For this review, take the finished solid that the model builds, in its own axes (mm). A direction names the side the tool comes from. Give positions to 0.01 mm unless a question says otherwise; leave off trailing zeros. Order: outer loops, then holes, each group sorted by start corner. A loop starts at its lowest first (then second) coordinate and runs counter-clockwise, first axis right, second up. Notation, with made-up numbers: (5, 25) - (30, 25) arc R19 cw to (30, 53) - close; hole circle Ø11 at (88, -4). An arc over 180 degrees is marked (long way). Answer as a JSON object with one key per item and string values. Group by question number.
from build123d import *

# Parameters (mm, degrees)
SKETCH1_W             = 30
SKETCH1_H             = 20
BOSS_EXTRUDE1_DEPTH   = 4
SKETCH2_R             = 4
BOSS_EXTRUDE2_DEPTH   = 3.5
M4X0_7_TAPPED_HOLE1_D = 3.3
SKETCH6_R             = 3
SKETCH6_R_2           = 1.65
BOSS_EXTRUDE3_DEPTH   = 0.5


with BuildPart() as part:
    # Sketch1 → Boss-Extrude1 (new body)
    with BuildSketch(Plane(origin=(0, 0, 0), x_dir=(1, 0, 0), z_dir=(0, 1, 0))):
        with Locations((9.74321034, 0)):
            Rectangle(SKETCH1_W, SKETCH1_H)
    extrude(amount=BOSS_EXTRUDE1_DEPTH)

    # Sketch2 → Boss-Extrude2 (add)
    with BuildSketch(Plane(origin=(0, 4, 0), x_dir=(1, 0, 0), z_dir=(0, 1, 0))):
        Circle(SKETCH2_R)
    extrude(amount=BOSS_EXTRUDE2_DEPTH)

    # M4x0.7 Tapped Hole1 (through all)
    with Locations(Plane(origin=(0, 0, 0), x_dir=(-1, 0, 0), z_dir=(0, -1, 0))):
        with Locations((0, 0)):
            Hole(M4X0_7_TAPPED_HOLE1_D / 2)

    # Sketch6 → Boss-Extrude3 (add)
    with BuildSketch(Plane(origin=(0, 7.5, 0), x_dir=(1, 0, 0), z_dir=(0, 1, 0))):
        Circle(SKETCH6_R)
        Circle(SKETCH6_R_2, mode=Mode.SUBTRACT)
    extrude(amount=BOSS_EXTRUDE3_DEPTH)


solid = part.part
1) For faces 1 (the face through (-0.867, 5.726, 3.905)), 2 (the face through (10, 0, 0)), list the 3-axis set-ups (+Z, -Z, +X, -X, +Y, -Y) from which the entire face can be reached by the end or side of a thin tool; tool diameter is ignored.
2) Consider section D-D (z = 2.25). Give the boundary of the cut face in (x, y).
3) Consider section A-A (z = 0). Give the boundary of the cut face in (x, y).
4) For line 1 (Z direction, x = 0, y = 3); line 2 (Z direction, x = 0, y = 7.8), list the stretches that pass through material, from the lowest coordinate up.
5) For pin 1 (2 mm diameter, centred on x = 0, z = 0, fed in from -Y); pin 2 (10 mm diameter, centred on x = 9.5, z = 2, fed in from +Y), all flat-tipped, find the tip position at first contact; note any pin that passes through.
6) Consider section B-B (x = 0). Give the boundary of the cut face in (y, z), plus the area to 3 significant figures.
7) Consider section C-C (y = 6.75). Give the boundary of the cut face in (x, z), plus the area to 3 significant figures.
Result set:
{
 "1": {"face 1": "+Y", "face 2": "+Z, -Z, +X, -X, -Y"},
 "2": {"outline": "(-5.26, 0) - (24.74, 0) - (24.74, 4) - (3.31, 4) - (3.31, 7.5) - (1.98, 7.5) - (1.98, 8) - (-1.98, 8) - (-1.98, 7.5) - (-3.31, 7.5) - (-3.31, 4) - (-5.26, 4) - close"},
 "3": {"outline": "(-5.26, 0) - (-1.65, 0) - (-1.65, 8) - (-3, 8) - (-3, 7.5) - (-4, 7.5) - (-4, 4) - (-5.26, 4) - close; (1.65, 0) - (24.74, 0) - (24.74, 4) - (4, 4) - (4, 7.5) - (3, 7.5) - (3, 8) - (1.65, 8) - close"},
 "4": {"line 1": "z = -10 to -1.65, 1.65 to 10", "line 2": "z = -3 to -1.65, 1.65 to 3"},
 "5": {"pin 1": "passes through", "pin 2": "stops at y = 4"},
 "6": {"outline": "(0, -10) - (4, -10) - (4, -4) - (7.5, -4) - (7.5, -3) - (8, -3) - (8, -1.65) - (0, -1.65) - close; (0, 1.65) - (8, 1.65) - (8, 3) - (7.5, 3) - (7.5, 4) - (4, 4) - (4, 10) - (0, 10) - close", "area": "84.6 mm2"},
 "7": {"outline": "circle Ø8 at (0, 0); hole circle Ø3.3 at (0, 0)", "area": "41.7 mm2"}
}
